Geometry: final body of the model. Coordinates: model frame, mm. Coordinates: 2 decimals unless noted, no trailing zeros. Write each loop counter-clockwise with the first axis right and the second up, starting at its lowest first coordinate (ties: lowest second). Pieces come first, ordered by that corner, then holes. Notation, with made-up numbers: (40, 24.5) - (76, 24.5) arc R20 ccw to (76, 51.5) - close; hole circle Ø2 at (-23.75, -3). An arc over 180 degrees is marked (long way). Answer as a JSON object with one key per item and string values. Group by question number.
Item 1: First-contact query: pin 1 Ø0.8 at (y, z) = (-44, 0.5) entering from -X; pin 2 Ø0.8 at (x, z) = (42, 0.5) entering from -Y; pin 3 Ø0.8 at (y, z) = (-44, 1) entering from +X. Flat tips, straight axial feed; report the tip coordinate or a pass-through.
Item 2: Section A-A on z = 1.15. State how many separate pieces and enclosed holes the cut face has, and give its area (3 significant figures).
Item 3: Line query: line 1 along Y through (x, z) = (28.67, 1.1) (3 decimals); line 2 along Y through (x, z) = (21, 0.65); line 3 along X through (y, z) = (39.6, 1.15) (3 decimals). Output: solid intervals per line, ascending. Write a range as from..to.
Item 4: Section B-B on x = -22. Return loops of the section in (y, z), and give its area (3 significant figures).
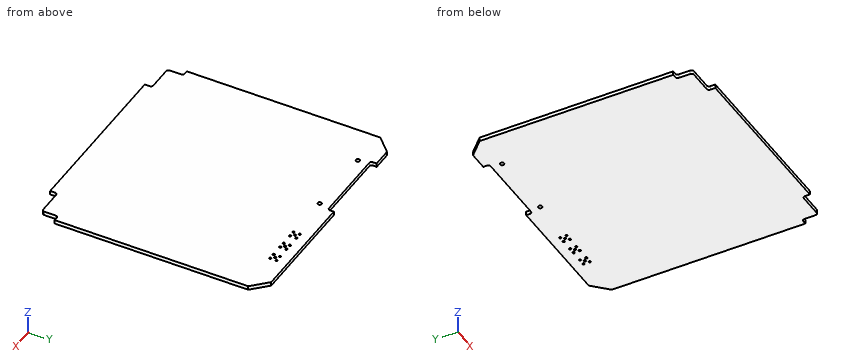
```python
from build123d import *

# Parameters (mm, degrees)
SKETCH1_R           = 0.425
SKETCH1_R_2         = 0.8
BOSS_EXTRUDE1_DEPTH = 1.6


with BuildPart() as part:
    # Sketch1 → Boss-Extrude1 (new body)
    with BuildSketch(Plane(origin=(0, 0, -0.0125), x_dir=(-1, 0, 0), z_dir=(0, 0, -1))):
        with BuildLine():
            Line((35.3, -50), (35.3, -48))
            ThreePointArc((35.3, -48), (35.592893219, -47.292893219), (36.3, -47))
            Line((36.3, -47), (45.8, -47))
            ThreePointArc((45.8, -47), (46.507106781, -46.707106781), (46.8, -46))
            Line((46.8, -46), (46.8, -41.4))
            ThreePointArc((46.8, -41.4), (47.092893219, -40.692893219), (47.8, -40.4))
            Line((47.8, -40.4), (49.3, -40.4))
            Line((49.3, -40.4), (49.3, 39.2))
            Line((49.3, 39.2), (43.2, 45.3))
            Line((43.2, 45.3), (35.500000002, 45.3))
            Line((35.500000002, 45.3), (35.500000002, 43.8))
            ThreePointArc((35.500000002, 43.8), (35.207106783, 43.092893219), (34.500000002, 42.8))
            Line((34.500000002, 42.8), (4.499999998, 42.8))
            ThreePointArc((4.499999998, 42.8), (3.792893217, 43.092893219), (3.499999998, 43.8))
            Line((3.499999998, 43.8), (3.499999998, 45.3))
            Line((3.499999998, 45.3), (-43.2, 45.3))
            Line((-43.2, 45.3), (-49.3, 39.2))
            Line((-49.3, 39.2), (-49.3, -40.4))
            Line((-49.3, -40.4), (-47.8, -40.4))
            ThreePointArc((-47.8, -40.4), (-47.092893219, -40.692893219), (-46.8, -41.4))
            Line((-46.8, -41.4), (-46.8, -46))
            ThreePointArc((-46.8, -46), (-46.507106781, -46.707106781), (-45.8, -47))
            Line((-45.8, -47), (-36.3, -47))
            ThreePointArc((-36.3, -47), (-35.592893219, -47.292893219), (-35.3, -48))
            Line((-35.3, -48), (-35.3, -50))
            Line((-35.3, -50), (35.3, -50))
        make_face()
        with Locations(Location((-21.27, 40.87, 0), (0, 0, 180))):
            Circle(SKETCH1_R, mode=Mode.SUBTRACT)
        with Locations(Location((-23.81, 40.87, 0), (0, 0, 180))):
            Circle(SKETCH1_R, mode=Mode.SUBTRACT)
        with Locations(Location((-22.54, 39.6, 0), (0, 0, 180))):
            Circle(SKETCH1_R, mode=Mode.SUBTRACT)
        with Locations(Location((-13.87, 40.87, 0), (0, 0, 180))):
            Circle(SKETCH1_R, mode=Mode.SUBTRACT)
        with Locations(Location((-23.81, 38.33, 0), (0, 0, 180))):
            Circle(SKETCH1_R, mode=Mode.SUBTRACT)
        with Locations(Location((-16.41, 40.87, 0), (0, 0, 180))):
            Circle(SKETCH1_R, mode=Mode.SUBTRACT)
        with Locations(Location((-15.14, 39.6, 0), (0, 0, 180))):
            Circle(SKETCH1_R, mode=Mode.SUBTRACT)
        with Locations(Location((-21.27, 38.33, 0), (0, 0, 180))):
            Circle(SKETCH1_R, mode=Mode.SUBTRACT)
        with Locations(Location((-28.67, 40.87, 0), (0, 0, 180))):
            Circle(SKETCH1_R, mode=Mode.SUBTRACT)
        with Locations(Location((-31.21, 40.87, 0), (0, 0, 180))):
            Circle(SKETCH1_R, mode=Mode.SUBTRACT)
        with Locations(Location((-16.41, 38.33, 0), (0, 0, 180))):
            Circle(SKETCH1_R, mode=Mode.SUBTRACT)
        with Locations(Location((-29.94, 39.6, 0), (0, 0, 180))):
            Circle(SKETCH1_R, mode=Mode.SUBTRACT)
        with Locations(Location((-31.21, 38.33, 0), (0, 0, 180))):
            Circle(SKETCH1_R, mode=Mode.SUBTRACT)
        with Locations(Location((-28.67, 38.33, 0), (0, 0, 180))):
            Circle(SKETCH1_R, mode=Mode.SUBTRACT)
        with Locations(Location((33.775, 38.54, 0), (0, 0, 180))):
            Circle(SKETCH1_R_2, mode=Mode.SUBTRACT)
        with Locations((5.225, 38.54)):
            Circle(SKETCH1_R_2, mode=Mode.SUBTRACT)
        with Locations(Location((-13.87, 38.33, 0), (0, 0, 180))):
            Circle(SKETCH1_R, mode=Mode.SUBTRACT)
    extrude(amount=-BOSS_EXTRUDE1_DEPTH)


solid = part.part
```
Checks:
{
 "1": {"pin 1": "x = -46.8", "pin 2": "y = -47", "pin 3": "x = 46.8"},
 "2": {"separate pieces": "1", "enclosed holes": "17", "area": "9,150 mm^2"},
 "3": {"line 1": "-50..37.905, 38.755..40.445, 41.295..45.3", "line 2": "-50..38, 38.66..40.54, 41.2..45.3", "line 3": "-48.9..14.715, 15.565..22.115, 22.965..29.515, 30.365..48.9"},
 "4": {"outline": "(-50, -0.01) - (42.8, -0.01) - (42.8, 1.59) - (-50, 1.59) - close", "area": "148 mm^2"}
}
